Part model, mm, in its own coordinate system. Coordinates: 2 decimals unless noted, no trailing zeros. Loops run counter-clockwise (first coordinate to the right, second up) from the corner with the lowest first, then second, coordinate; pieces in that order, holes last. Notation, with made-up numbers: M -38,-20.5 L 19,-20.5 A10 ccw 19,-15.5 Z; hole C -35,-27.5 d11. An arc over 180 degrees is marked long. Use CSV: the item, a comma, the result in double quotes. Start each with the question number.
from build123d import *

# Parameters (mm, degrees)
SKETCH1_W           = 450
SKETCH1_H           = 420
SKETCH1_W_2         = 430
SKETCH1_H_2         = 400
BOSS_EXTRUDE1_DEPTH = 10
BOSS_EXTRUDE2_DEPTH = 10
SKETCH8_W           = 11.547005384
SKETCH8_H           = 10
BOSS_EXTRUDE3_DEPTH = 10.67
SKETCH9_R           = 5.335
BOSS_EXTRUDE4_DEPTH = 12.7
SKETCH10_R          = 5.335
BOSS_EXTRUDE5_DEPTH = 12.7


with BuildPart() as part:
    # Sketch1 → Boss-Extrude1 (new body)
    with BuildSketch(Plane(origin=(0, 0, 0), x_dir=(1, 0, 0), z_dir=(0, 1, 0))):
        Rectangle(SKETCH1_W, SKETCH1_H)
        Rectangle(SKETCH1_W_2, SKETCH1_H_2, mode=Mode.SUBTRACT)
    extrude(amount=BOSS_EXTRUDE1_DEPTH)

    # Sketch4 → Boss-Extrude2 (add)
    with BuildSketch(Plane.XY.offset(210)):
        Polygon((-225, 0), (-109.529946162, -200), (-97.982940778, -200), (-213.452994616, 0), align=None)
        Polygon((225, 0), (340.470053838, -200), (328.923048454, -200), (213.452994616, 0), align=None)
    boss_extrude2 = extrude(amount=-BOSS_EXTRUDE2_DEPTH)

    # Mirror1: Boss-Extrude2 across plane
    add(boss_extrude2.mirror(Plane.XY))

    # Sketch8 → Boss-Extrude3 (add)
    with BuildSketch(Plane.XZ.offset(200)):
        with Locations((-103.75644347, 205)):
            Rectangle(SKETCH8_W, SKETCH8_H)
        with Locations((334.696551146, 205)):
            Rectangle(SKETCH8_W, SKETCH8_H)
    boss_extrude3 = extrude(amount=BOSS_EXTRUDE3_DEPTH)

    # Mirror2: Boss-Extrude3 across plane
    add(boss_extrude3.mirror(Plane.XY))

    # Sketch9 → Boss-Extrude4 (add)
    with BuildSketch(Plane.ZY.offset(109.529946162)):
        with Locations(Location((205.028494261, -205.335, 0), (0, 0, 199.516018921))):
            Circle(SKETCH9_R)
    boss_extrude4 = extrude(amount=BOSS_EXTRUDE4_DEPTH)

    # Sketch10 → Boss-Extrude5 (add)
    with BuildSketch(Plane.ZY.offset(-328.923048454)):
        with Locations(Location((205, -205.335, 0), (0, 0, 159.587697496))):
            Circle(SKETCH10_R)
    boss_extrude5 = extrude(amount=BOSS_EXTRUDE5_DEPTH)

    # Mirror3: Boss-Extrude4, Boss-Extrude5 across plane
    add(boss_extrude4.mirror(Plane.XY))
    add(boss_extrude5.mirror(Plane.XY))


solid = part.part
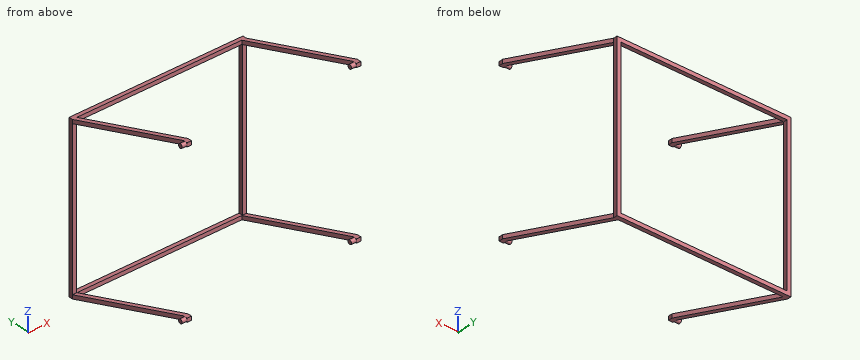
1. Wall check: probe 1 along Y at (x, z) = (221.5, -17.5). Give the ranges that are in metal, low to high.
2. Slice it at B-B, the plane z = 160. List the corners of the cut face in (x, y), and give its area (3 significant figures).
3. Pin check, flat tips, straight feed: pin 1 (3 mm diameter, centred on y = -201.5, z = 206.5, fed in from -X); pin 2 (5 mm diameter, centred on x = -218.5, z = 28.5, fed in from -Y). Stop position of each tip, or through.
4. Slice it at A-A, the plane x = 173. List the corners of the cut face in (y, z), and give its area (3 significant figures).
5. Slice it at C-C, the plane y = -118. List the corners of the cut face in (x, z).
Found:
1,probe 1,"0 to 10"
2,outline,"M -225,0 L -215,0 L -215,10 L -225,10 Z; M 215,0 L 225,0 L 225,10 L 215,10 Z"
2,area,"200 mm^2"
3,pin 1,"x = -122.23"
3,pin 2,"y = 0"
4,outline,"M 0,-210 L 10,-210 L 10,-200 L 0,-200 Z; M 0,200 L 10,200 L 10,210 L 0,210 Z"
4,area,"200 mm^2"
5,outline,"M -156.87,-210 L -145.33,-210 L -145.33,-200 L -156.87,-200 Z; M -156.87,200 L -145.33,200 L -145.33,210 L -156.87,210 Z; M 281.58,-210 L 293.13,-210 L 293.13,-200 L 281.58,-200 Z; M 281.58,200 L 293.13,200 L 293.13,210 L 281.58,210 Z"
